Geometry check sheet. Reference: the model listing, model coordinates, mm. A direction names the side the tool comes from. Give positions to 0.01 mm unless a question says otherwise; leave off trailing zeros. Loops run counter-clockwise (first coordinate to the right, second up) from the corner with the lowest first, then second, coordinate; pieces in that order, holes last. Notation, with made-up numbers: (63.25, 52) -> (85.25, 52) arc R16 cw to (85.25, 81) -> close; hole circle Ø10 at (27, 70.5). An arc over 180 degrees is marked (long way). One line per item, written item: value. Start each with the question number.
(1) Tool access check on faces 1 (the face through (7.847, 25, 31)), 2 (the face through (53, 20, 25)), 3 (the face through (41, 7.722, 31)), 4 (the face through (52.2, 15, 25)). Record the directions out of +Z, -Z, +X, -X, +Y, -Y that give a thin tool (end or side, any length) a straight path to the whole face; none if there is none.
(2) Draft check along Y on faces 5 (the face through (6, 27.2, 31)), 6 (the face through (51.661, 15, 31)), 7 (the face through (53, 15, 21)). Enter one of: pulls with the +Y half, pulls with the -Y half, needs draft (parallel to the pull), parting line crosses it, or undercut.
(3) Gauge pin test, flat ends, axial feed: pin 1 Ø0.6 at (x, z) = (36, 30.5) entering from +Y; pin 2 Ø8 at (x, y) = (22, 6.5) entering from -Z; pin 3 Ø4 at (y, z) = (15.5, 22) entering from -X. Record the tip position at first contact, or that the pin passes through.
(4) Sectioned sample at A-A, the plane x = 40.5. Record the cut outline in (y, z).
(5) Sectioned sample at B-B, the plane y = 20.5. Record the cut outline in (x, z).
(6) Sectioned sample at D-D, the plane y = 13.75. Record the cut outline in (x, z).
(7) Scan lines: line 1 along Z through (x, y) = (23, 12.75); line 2 along X through (y, z) = (18.5, 23.25). Record each from-to range of solid material in increasing order. Write a range as from..to.
(8) Sectioned sample at C-C, the plane z = 30.5. Record the cut outline in (x, y).
from build123d import *

# Parameters (mm, degrees)
BOX011_W     = 1.5
BOX011_H     = 10
BOX011_DEPTH = 9
BOX010_W     = 51.8
BOX010_H     = 25.2
BOX010_DEPTH = 2
CHAMFER_SIZE = 3
SKETCH_W     = 21.634724
SKETCH_H     = 14.706005
SKETCH_W_2   = 39.946578
SKETCH_H_2   = 4.737023
POCKET_DEPTH = 3


with BuildPart() as obj1:
    # Box011 → Box011 (new body)
    with BuildSketch(Plane(origin=(52.2, 10, 21), x_dir=(1, 0, 0), z_dir=(0, 0, 1))):
        with Locations((0.75, 5)):
            Rectangle(BOX011_W, BOX011_H)
    extrude(amount=BOX011_DEPTH)


with BuildPart() as bat_controller_sep:
    # Box010 → Box010 (new body)
    with BuildSketch(Plane(origin=(2, 2, 30), x_dir=(1, 0, 0), z_dir=(0, 0, 1))):
        with Locations((25.9, 12.6)):
            Rectangle(BOX010_W, BOX010_H)
    extrude(amount=BOX010_DEPTH)

    # Chamfer
    chamfer_edges = [bat_controller_sep.edges().sort_by_distance(p)[0] for p in [
        (2, 2, 31),
        (2, 27.2, 31),
        (53.8, 2, 31),
        (53.8, 27.2, 31),
    ]]
    chamfer(chamfer_edges, length=CHAMFER_SIZE)

    # Sketch (on Face5 of Chamfer) → Pocket (cut)
    with BuildSketch(Plane(origin=(0, 0, 30), x_dir=(1, 0, 0), z_dir=(0, 0, -1))):
        with Locations((40.844102, -15.075252)):
            Rectangle(SKETCH_W, SKETCH_H)
        with Locations((27.819974, -24.837604)):
            Rectangle(SKETCH_W_2, SKETCH_H_2)
    extrude(amount=-POCKET_DEPTH, mode=Mode.SUBTRACT)

    # Fusion008: union obj1
    add(obj1.part)


solid = bat_controller_sep.part
Calculated:
1. face 1: +Z, -Z, +Y
1. face 2: -Z, +X, -X, +Y
1. face 3: +Z, -Z
1. face 4: -Z, -X, +Y, -Y
2. face 5: pulls with the +Y half
2. face 6: undercut
2. face 7: needs draft
3. pin 1: stops at y = 22.47
3. pin 2: stops at z = 30
3. pin 3: stops at x = 52.2
4. outline: (2, 30) -> (7.72, 30) -> (7.72, 32) -> (2, 32) -> close; (22.43, 30) -> (22.47, 30) -> (22.47, 32) -> (22.43, 32) -> close
5. outline: (2, 30) -> (30.03, 30) -> (30.03, 32) -> (2, 32) -> close; (51.66, 30) -> (53.8, 30) -> (53.8, 32) -> (51.66, 32) -> close
6. outline: (2, 30) -> (30.03, 30) -> (30.03, 32) -> (2, 32) -> close; (51.66, 30) -> (52.2, 30) -> (52.2, 21) -> (53.7, 21) -> (53.7, 30) -> (53.8, 30) -> (53.8, 32) -> (51.66, 32) -> close
7. line 1: z = 30..32
7. line 2: x = 52.2..53.7
8. outline: (2, 5) -> (5, 2) -> (50.8, 2) -> (53.8, 5) -> (53.8, 24.2) -> (50.8, 27.2) -> (47.79, 27.2) -> (47.79, 22.47) -> (7.85, 22.47) -> (7.85, 27.2) -> (5, 27.2) -> (2, 24.2) -> close; hole (30.03, 7.72) -> (51.66, 7.72) -> (51.66, 22.43) -> (30.03, 22.43) -> close
